Geometry check sheet. Reference: the model listing, model coordinates, mm. Round coordinates to 2 decimals unless told otherwise and drop trailing zeros. Write each loop counter-clockwise with the first axis right and the second up, starting at its lowest first coordinate (ties: lowest second). Pieces come first, ordered by that corner, then holes. Notation, with made-up numbers: M 42.25,41 L 64.25,41 A34 cw 64.25,80 Z; hole C 15.5,-21 d7. An arc over 180 degrees is marked long. Answer as CSV lines item,"result". Start each with the question number.
```python
from build123d import *

# Parameters (mm, degrees)
SKETCH1_R           = 3
BOSS_EXTRUDE1_DEPTH = 70
SKETCH2_R           = 5.8
BOSS_EXTRUDE2_DEPTH = 4.3
FILLET1_R           = 1


with BuildPart() as part:
    # Sketch1 → Boss-Extrude1 (new body)
    with BuildSketch(Plane(origin=(0, 0, 0), x_dir=(1, 0, 0), z_dir=(0, 1, 0))):
        with Locations(Location((0, 0, 0), (0, 0, 270))):  # turned: the seam where the file's is
            Circle(SKETCH1_R)
    extrude(amount=BOSS_EXTRUDE1_DEPTH)

    # Sketch2 → Boss-Extrude2 (add)
    with BuildSketch(Plane(origin=(0, 70, 0), x_dir=(1, 0, 0), z_dir=(0, 1, 0))):
        with Locations(Location((0, 0, 0), (0, 0, 270))):  # turned: the seam where the file's is
            Circle(SKETCH2_R)
    extrude(amount=BOSS_EXTRUDE2_DEPTH)

    # Fillet1
    fillet1_edges = [part.edges().sort_by_distance(p)[0] for p in [
        (0, 70, -5.8),
        (0, 74.3, -5.8),
    ]]
    fillet(fillet1_edges, radius=FILLET1_R)


solid = part.part
```
1) Section check C-C, the plane y = 66. Record the cut outline in (x, z), plus the area to 3 significant figures.
2) Go/stop test with flat-tipped pins: pin 1 (2 mm diameter, centred on y = 27, z = 4.5, fed in from -X); pin 2 (4 mm diameter, centred on x = -4, y = 51, fed in from -Z); pin 3 (2 mm diameter, centred on x = -3.5, z = -4, fed in from -Y); pin 4 (4 mm diameter, centred on x = 0.5, y = 39.5, fed in from -Z). Record where each tip stops, or that it passes through.
3) Section check A-A, the plane z = 0. Record the cut outline in (x, y), plus the area to 3 significant figures.
4) Section check B-B, the plane x = 0. Record the cut outline in (y, z).
5) Scan lines: line 1 (Y direction, x = -4, z = 0.25); line 2 (X direction, y = 50, z = 0); line 3 (Y direction, x = 4.75, z = 2). Record each from-to range of solid material in increasing order. Write a range as from..to.
6) Mould release check, pull along Y, two halves, no side actions. Record for faces 1 (the flat face through (0, 74.3, 0)), 2 (the flat face through (0, 0, 0)), 3 (the cylindrical face through (0.255, 72.134, -5.794)): released by +Y, released by -Y, zero draft, split by the parting line, or undercut.
Results:
1,outline,"C 0,0 d6"
1,area,"28.3 mm^2"
2,pin 1,"passes through"
2,pin 2,"stops at z = -2.24"
2,pin 3,"stops at y = 70"
2,pin 4,"stops at z = -3"
3,outline,"M -5.8,71 A1 ccw -4.8,70 L -3,70 L -3,0 L 3,0 L 3,70 L 4.8,70 A1 ccw 5.8,71 L 5.8,73.3 A1 ccw 4.8,74.3 L -4.8,74.3 A1 ccw -5.8,73.3 Z"
3,area,"469 mm^2"
4,outline,"M 0,-3 L 70,-3 L 70,-4.8 A1 ccw 71,-5.8 L 73.3,-5.8 A1 ccw 74.3,-4.8 L 74.3,4.8 A1 ccw 73.3,5.8 L 71,5.8 A1 ccw 70,4.8 L 70,3 L 0,3 Z"
5,line 1,"y = 70..74.3"
5,line 2,"x = -3..3"
5,line 3,"y = 70.06..74.24"
6,face 1,"released by +Y"
6,face 2,"released by -Y"
6,face 3,"zero draft"
